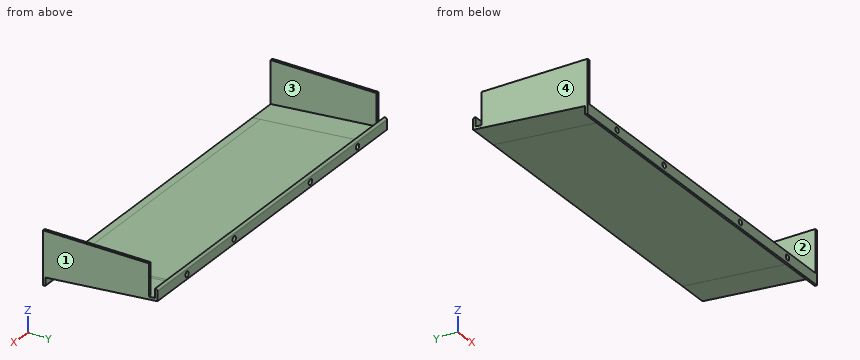
from build123d import *

# Parameters (mm, degrees)
EXTRUDE_1_DEPTH     = 165
SKETCH_2_R          = 1.5
CUT_EXTRUDE_2_DEPTH = 66
EXTRUDE_2_DEPTH     = 1.5
EXTRUDE_START       = 17.5
EXTRUDE_3_DEPTH     = 17.5
EXTRUDE_4_DEPTH     = 1.5
CUT_EXTRUDE_3_DEPTH = 1.5


with BuildPart() as part:
    # 草图1 → 凸台-拉伸1 (new body)
    with BuildSketch(Plane(origin=(0, 0, 0), x_dir=(0, 0, -1), z_dir=(1, 0, 0))):
        with BuildLine():
            Line((0, 4.49026118), (5.69, -54.13973882))
            Line((5.69, -54.13973882), (6.125751322, -58.62973882))
            Line((6.125751322, -58.62973882), (12.125751322, -58.62973882))
            Line((12.125751322, -58.62973882), (12.125751322, -57.62973882))
            ThreePointArc((12.125751322, -57.62973882), (11.979304712, -57.27618543), (11.625751322, -57.12973882))
            Line((11.625751322, -57.12973882), (7.487224752, -57.12973882))
            Line((7.487224752, -57.12973882), (7.05147343, -52.63973882))
            Line((7.05147343, -52.63973882), (1.393781374, 5.657358767))
            Line((1.393781374, 5.657358767), (1.370240908, 5.899920726))
            ThreePointArc((1.370240908, 5.899920726), (1.337917334, 5.964308309), (1.270708535, 5.99026118))
            Line((1.270708535, 5.99026118), (-4, 5.99026118))
            ThreePointArc((-4, 5.99026118), (-4.707106781, 5.697367961), (-5, 4.99026118))
            Line((-5, 4.99026118), (-5, 4.49026118))
            Line((-5, 4.49026118), (0, 4.49026118))
        make_face()
    extrude(amount=EXTRUDE_1_DEPTH)

    # 草图2 → 切除-拉伸2 (cut)
    with BuildSketch(Plane(origin=(0, 5.99026118, 0), x_dir=(1, 0, 0), z_dir=(0, 1, 0))):
        with Locations(Location((156.807985478, -1.364645732, 0), (0, 0, 270))):
            Circle(SKETCH_2_R)
        with Locations(Location((115.749974851, -1.364645732, 0), (0, 0, 270))):
            Circle(SKETCH_2_R)
        with Locations(Location((49.250025149, -1.364645732, 0), (0, 0, 65.47273381))):
            Circle(SKETCH_2_R)
        with Locations(Location((8.192014522, -1.364645732, 0), (0, 0, 65.47273381))):
            Circle(SKETCH_2_R)
        with Locations(Location((8.192014522, 9.011696347, 0), (0, 0, 270))):
            Circle(SKETCH_2_R)
        with Locations(Location((156.807985478, 9.011696347, 0), (0, 0, 270))):
            Circle(SKETCH_2_R)
        with Locations(Location((115.749974851, 9.011696347, 0), (0, 0, 270))):
            Circle(SKETCH_2_R)
        with Locations(Location((49.250025149, 9.011696347, 0), (0, 0, 270))):
            Circle(SKETCH_2_R)
    extrude(amount=-CUT_EXTRUDE_2_DEPTH, mode=Mode.SUBTRACT)

    # 草图3 → 凸台-拉伸2 (add)
    with BuildSketch(Plane(origin=(165, 0, 0), x_dir=(0, 0, -1), z_dir=(1, 0, 0))):
        Polygon((0.32961608, 1.093883189), (-17.67038392, 1.093883189), (-17.67038392, -58.62973882), (6.125751322, -58.62973882), align=None)
    extrude(amount=-EXTRUDE_2_DEPTH)

    # 草图5 → 凸台-拉伸3 (add)
    with BuildSketch(Plane.ZY.offset(EXTRUDE_START)):
        with BuildLine():
            Line((4, 5.99026118), (-1.270708535, 5.99026118))
            ThreePointArc((-1.270708535, 5.99026118), (-1.337917334, 5.964308309), (-1.370240908, 5.899920726))
            Line((-1.370240908, 5.899920726), (-7.487224752, -57.12973882))
            Line((-7.487224752, -57.12973882), (-11.625751322, -57.12973882))
            ThreePointArc((-11.625751322, -57.12973882), (-11.979304712, -57.27618543), (-12.125751322, -57.62973882))
            Line((-12.125751322, -57.62973882), (-12.125751322, -58.62973882))
            Line((-12.125751322, -58.62973882), (-6.125751322, -58.62973882))
            Line((-6.125751322, -58.62973882), (0, 4.49026118))
            Line((0, 4.49026118), (5, 4.49026118))
            Line((5, 4.49026118), (5, 4.99026118))
            ThreePointArc((5, 4.99026118), (4.707106781, 5.697367961), (4, 5.99026118))
        make_face()
    extrude_3 = extrude(amount=-EXTRUDE_3_DEPTH)

    # 镜向2: 凸台-拉伸3 across plane
    add(extrude_3.mirror(Plane(origin=(82.5, 0, 0), x_dir=(0, 0, 1), z_dir=(1, 0, 0))))

    # 草图6 → 凸台-拉伸4 (add)
    with BuildSketch(Plane(origin=(182.5, 0, 0), x_dir=(0, 0, -1), z_dir=(1, 0, 0))):
        Polygon((0.32961608, 1.093883189), (-17.67038392, 1.093883189), (-17.67038392, -58.62973882), (6.125751322, -58.62973882), align=None)
    extrude_4 = extrude(amount=-EXTRUDE_4_DEPTH)

    # 草图7 → 切除-拉伸3 (cut)
    with BuildSketch(Plane(origin=(165, 0, 0), x_dir=(0, 0, -1), z_dir=(1, 0, 0))):
        Polygon((0.32961608, 1.093883189), (6.382938613, -61.279807515), (-18.871026255, -61.279807515), (-18.871026255, 1.093883189), align=None)
    extrude(amount=-CUT_EXTRUDE_3_DEPTH, mode=Mode.SUBTRACT)

    # 镜向4: 凸台-拉伸4 across plane
    add(extrude_4.mirror(Plane(origin=(82.5, 0, 0), x_dir=(0, 0, 1), z_dir=(1, 0, 0))))


solid = part.part
Input: part model. Units: mm. Frame: model coordinates. Face numbers are marked on the shaded views. Round coordinates to 2 decimals unless told otherwise and drop trailing zeros. Loops run counter-clockwise (first coordinate to the right, second up) from the corner with the lowest first, then second, coordinate; pieces in that order, holes last. Notation, with made-up numbers: M 73,60 L 99,60 A20 cw 99,74 Z; hole C 4,4 d4. An arc over 180 degrees is marked long. Answer as CSV lines item,"result". Start each with the question number.
(1) Line query: line 1 (X direction, y = -42, z = 5.5); line 2 (Y direction, x = 65, z = 3); line 3 (Z direction, x = 72, y = -26). Output: solid intervals per line, ascending. Write a range as [from, to].
(2) Draft query along X for the marked faces 1, 2, 3 and 4. Return one class per face: released by +X, released by -X, zero draft, split by the parting line, or undercut.
(3) Section B-B, the plane x = 21. Output: boundary loops of the cut face in (y, z).
(4) Section A-A, the plane z = 8. Output: boundary loops of the cut face in (x, y), plus the area to 3 significant figures.
(5) Section C-C, the plane y = -42. Output: boundary loops of the cut face in (x, z).
(6) Section D-D, the plane y = -2. Output: boundary loops of the cut face in (x, z).
(7) First-contact query: pin 1 (8 mm diameter, centred on x = 123, y = -44, fed in from -Z); pin 2 (1.5 mm diameter, centred on x = 151.5, y = -48, fed in from +Z); pin 3 (3 mm diameter, centred on x = 18, y = -33, fed in from -Z); pin 4 (1.8 mm diameter, centred on x = 156.81, z = 1.36, fed in from +Y). Flat tips, straight axial feed; report the tip coordinate or a pass-through.
Values found:
1,line 1,"x = [-17.5, -16], [181, 182.5]"
1,line 2,"y = [4.49, 5.99]"
1,line 3,"z = [-4.47, -2.96]"
2,face 1,"released by +X"
2,face 2,"undercut"
2,face 3,"undercut"
2,face 4,"released by -X"
3,outline,"M -58.63,-12.13 L -57.63,-12.13 A0.5 ccw -57.13,-11.63 L -57.13,-7.49 L 5.9,-1.37 A0.1 ccw 5.99,-1.27 L 5.99,4 A1 ccw 4.99,5 L 4.49,5 L 4.49,0 L -58.63,-6.13 Z"
4,outline,"M -17.5,-58.63 L -16,-58.63 L -16,1.09 L -17.5,1.09 Z; M 181,-58.63 L 182.5,-58.63 L 182.5,1.09 L 181,1.09 Z"
4,area,"179 mm²"
5,outline,"M -17.5,-6.02 L 182.5,-6.02 L 182.5,17.67 L 181,17.67 L 181,-4.51 L -16,-4.51 L -16,17.67 L -17.5,17.67 Z"
6,outline,"M -17.5,-2.14 L 182.5,-2.14 L 182.5,17.67 L 181,17.67 L 181,-0.63 L -16,-0.63 L -16,17.67 L -17.5,17.67 Z"
7,pin 1,"stops at z = -6.6"
7,pin 2,"stops at z = -5.02"
7,pin 3,"stops at z = -5.29"
7,pin 4,"passes through"
